Check sheet for the modelled part. Datum: model origin and axes. Units: mm. A direction names the side the tool comes from. Coordinates: 2 decimals unless noted, no trailing zeros. Write each loop counter-clockwise with the first axis right and the second up, starting at its lowest first coordinate (ties: lowest second). Pieces come first, ordered by that corner, then holes. Notation, with made-up numbers: (78.25, -3.5) - (135.25, -3.5) arc R8 ccw to (135.25, 8.5) - close; hole circle Ø3 at (25.25, -27). An arc over 180 degrees is marked (long way). Answer as CSV lines item,"result". Start each with the question number.
Autodesk Inventor part; units mm, degrees
ref_plane "Work Plane1" through (-73, 67.0488, 53) normal (0, -0.2132164, 0.977005) x (1, 0, 0)
ref_plane "YZ Plane" through (0, 0, 0) normal (1, 0, 0) x (0, 1, 0)
ref_plane "XZ Plane" through (0, 0, 0) normal (0, 1, 0) x (-1, 0, 0)
sketch "Sketch1" plane through (0, 0, 0) normal (0, 0, 1) x (1, 0, 0)
  line L0 (-75, 67.0488) -> (75, 67.0488)
  arc A0 (-75, -67.9512) -> (-48.2091, -125.4046) centre (0, -67.9512) ccw
  arc A1 (48.2091, -125.4046) -> (75, -67.9512) centre (0, -67.9512) ccw
  arc A2 (32.1394, -106.2534) -> (-32.1394, -106.2534) centre (0, -67.9512) ccw
  line L1 (-48.2091, -125.4046) -> (-32.1394, -106.2534) construction
  line L2 (-32.1394, -106.2534) -> (0, -67.9512) construction
  line L3 (-48.2091, -125.4046) -> (-32.1394, -106.2534) construction
  line L4 (75, -67.9512) -> (75, 67.0488)
  line L5 (-75, -67.9512) -> (-75, 67.0488)
  line L6 (0, -67.9512) -> (0, -148.7803) construction
  line L7 (-32.1394, -106.2534) -> (-48.2091, -125.4046)
  line L8 (48.2091, -125.4046) -> (32.1394, -106.2534)
  point P0 (0, 0)
  dimension "d0" = 150
  dimension "d2" = 135
  dimension "d3" = 135
  dimension "d7" = 135
  dimension "d8" = 50
  dimension "d19" = 75
  dimension "d25" = 75
  dimension "d26" = 0
  dimension "d29" = 50
  dimension "d31" = 50
  dimension "d34" = 40
  dimension "d35" = 40
extrude "Extrusion1" add sketch "Sketch1" along normal blind 3
sketch "Sketch5" plane through (0, 0, 3) normal (0, 0, 1) x (1, 0, 0)
  arc A0 (32.1394, -106.2534) -> (-32.1394, -106.2534) centre (0, -67.9512) ccw
  line L0 (32.1394, -106.2534) -> (48.2091, -125.4046)
  line L1 (-48.2091, -125.4046) -> (-32.1394, -106.2534)
  arc A1 (37.2817, -112.3818) -> (-37.2817, -112.3818) centre (0, -67.9512) ccw
  arc A2 (32.1394, -106.2534) -> (-32.1394, -106.2534) centre (0, -67.9512) ccw
  arc A3 (32.1394, -106.2534) -> (-32.1394, -106.2534) centre (0, -67.9512) ccw
  arc A4 (41.7812, -117.7441) -> (-41.7812, -117.7441) centre (0, -67.9512) ccw
  arc A5 (46.2807, -123.1064) -> (-46.2807, -123.1064) centre (0, -67.9512) ccw
  line L2 (-46.2807, -123.1064) -> (-41.7812, -117.7441)
  line L3 (-37.2817, -112.3818) -> (-32.1394, -106.2534)
  line L4 (32.1394, -106.2534) -> (37.2817, -112.3818)
  line L5 (41.7812, -117.7441) -> (46.2807, -123.1064)
  point P0 (0, 0)
  dimension "d49" = 58
  dimension "d52" = 65
  dimension "d53" = 72
extrude "Extrusion3" add sketch "Sketch5" along normal blind 8 contours A0 L1 A1 L0 | A4 L1 A5 L0
sketch "Sketch7" plane through (-48.2091, -125.4046, 3) normal (0.7660444, -0.6427876, 0) x (0, 0, -1)
  line L0 (0, 10) -> (-8, 10)
  line L1 (-4.5, 10) -> (0, 10)
  line L2 (0, 10) -> (0, 17)
  line L3 (0, 10) -> (0, 17)
  line L4 (0, 17) -> (-4.5, 17)
  line L5 (0, 17) -> (-8, 17)
  arc A0 (-4.5, 10) -> (-4.5, 17) centre (-4.5, 13.5) ccw
  line L6 (-19.076, 75) -> (19.2246, 75) construction
  point P0 (3, 127.0537)
  dimension "d58" = 4.5
  dimension "d59" = 0
  dimension "d60" = 0
  dimension "d61" = 3.5
  dimension "d62" = 58
revolve "Revolution1" add sketch "Sketch7" angle 280 about axis through (0, -67.9512, 22.076) along (0, 0, -1)
sketch "Sketch18" plane through (0, 0, 0) normal (0, 0, -1) x (-1, 0, 0)
  arc A0 (32.1394, -106.2534) -> (-32.1394, -106.2534) centre (0, -67.9512) ccw
  line L0 (32.1394, -106.2534) -> (48.2091, -125.4046)
  arc A1 (32.1394, -106.2534) -> (-32.1394, -106.2534) centre (0, -67.9512) ccw
  line L1 (-32.1394, -106.2534) -> (-47.5756, -125.4046)
  line L2 (32.1394, -106.2534) -> (48.2091, -125.4046)
  line L3 (75, 67.0488) -> (-75, 67.0488)
  line L4 (-75, 67.0488) -> (-75, -67.9512)
  arc A2 (-75, -67.9512) -> (-48.2091, -125.4046) centre (0, -67.9512) ccw
  line L5 (-48.2091, -125.4046) -> (-32.1394, -106.2534)
  arc A3 (32.1394, -106.2534) -> (-32.1394, -106.2534) centre (0, -67.9512) ccw
  line L6 (32.1394, -106.2534) -> (48.2091, -125.4046)
  arc A4 (48.2091, -125.4046) -> (75, -67.9512) centre (0, -67.9512) ccw
  line L7 (75, -67.9512) -> (75, 67.0488)
  arc A5 (-75, -67.9512) -> (-48.2091, -125.4046) centre (0, -67.9512) ccw
  line L8 (-75, -67.9512) -> (-75, 67.0488)
  line L9 (75, -67.9512) -> (75, 67.0488)
  line L10 (75, 67.0488) -> (75, -67.9512)
  arc A6 (-75, -67.9512) -> (-48.2091, -125.4046) centre (0, -67.9512) ccw
  arc A7 (48.2091, -125.4046) -> (75, -67.9512) centre (0, -67.9512) ccw
  arc A8 (48.2091, -125.4046) -> (75, -67.9512) centre (0, -67.9512) ccw
  arc A9 (35.4639, -107.3379) -> (-35.4639, -107.3379) centre (0, -67.9512) ccw
  line L11 (0, -67.9512) -> (35.4639, -107.3379) construction
  line L12 (0, -67.9512) -> (-35.4639, -107.3379) construction
  line L13 (0, -67.9512) -> (0, -163.7516) construction
  arc A10 (46.2807, -123.1064) -> (-46.2807, -123.1064) centre (0, -67.9512) ccw construction
  line L14 (72, -67.9512) -> (72, 64.0488)
  line L15 (72, 64.0488) -> (-72, 64.0488)
  line L16 (-72, 64.0488) -> (-72, -67.9512)
  arc A11 (-72, -67.9512) -> (-48.1774, -121.4576) centre (0, -67.9512) ccw
  arc A12 (48.1774, -121.4576) -> (72, -67.9512) centre (0, -67.9512) ccw
  line L17 (-48.1774, -121.4576) -> (-35.4639, -107.3379)
  line L18 (35.4639, -107.3379) -> (48.1774, -121.4576)
  point P0 (0, 0)
  dimension "d99" = 84
  dimension "d100" = 42
  dimension "d101" = 53
  dimension "d102" = 3
  dimension "d103" = 3
extrude "Extrusion8" add sketch "Sketch18" against normal blind 53
sketch "Sketch19" plane through (75, -67.9512, 0) normal (1, 0, 0) x (0, 0, -1)
  line L0 (-3, 132) -> (-3, 0)
  line L1 (-3, 0) -> (-3, 0)
  line L2 (-3, 0) -> (-3, 132)
  line L3 (-11, 0) -> (-11, -53.5064)
  line L4 (-53, 0) -> (-53, 135)
  line L5 (-53, 0) -> (-53, -57.4533)
  line L6 (0, -57.4533) -> (-53, -57.4533)
  line L7 (-53, 135) -> (-53, -57.4533)
  line L8 (-53, -57.4533) -> (-11, -57.4533)
  line L9 (0, 135) -> (-53, 135)
  line L10 (-11, -57.4533) -> (-53, 135)
  point P0 (0, 67.9512)
  dimension "d106" = 0
extrude "Extrusion9" cut sketch "Sketch19" against normal blind 150
sketch "Sketch20" plane through (-32.1394, -106.2534, 15.1794) normal (0.7660444, -0.6427876, 0) x (0, 0, -1)
  ellipse E0 centre (7.6794, -11.4625) end of major axis (11.1794, -11.4625) minor radius 3.4979 (7.6794, -14.9604) -> (7.6794, -7.9647) ccw
  circle A0 centre (7.6794, -11.4625) radius 3.5
  line L0 (-25.5689, 50.0375) -> (41.9904, 50.0375) construction
  point P0 (15.1794, 102.0537)
  dimension "d109" = 61.5
revolve "Revolution4" cut sketch "Sketch20" angle 2 about axis through (0.0241, -67.9225, 40.7483) along (0, 0, -1)
mirror "Mirror3" about plane through (0, 0, 0) normal (1, 0, 0) of "Revolution4"
fillet "Fillet1" radius 2 12 edges at (75, 67.0488, 26.5) (-48.2091, -125.4046, 5.5) (-32.1394, -106.2534, 7.5897) (48.2091, -125.4046, 5.5) (32.1394, -106.2534, 7.5897) (-75, 67.0488, 26.5) (0, 67.0488, 0) (-67.9731, -99.6476, 0) (-75, -0.4512, 0) (67.9731, -99.6476, 0) (75, -0.4512, 0) (0, -17.9512, 0)
sketch "Sketch23" plane through (0, 0, 0) normal (0, 0, -1) x (-1, 0, 0)
  arc A0 (43.4935, -116.2556) -> (-43.4935, -116.2556) centre (0, -67.9512) ccw
  line L0 (0, -67.9512) -> (0, -128.8082) construction
  arc A1 (43.4935, -116.2556) -> (-43.4935, -116.2556) centre (0, -67.9512) ccw
  line L1 (-56.2917, -100.4512) -> (-50.2295, -96.9512) construction
  line L2 (0, -67.9512) -> (-50.2295, -96.9512) construction
  line L3 (-56.2917, -100.4512) -> (0, -67.9512) construction
  circle A2 centre (-55.0106, -95.6701) radius 3.5 construction
  line L4 (-59.6154, -93.8549) -> (-53.1953, -91.0653) construction
  arc A3 (38.8096, -111.0536) -> (-38.8096, -111.0536) centre (0, -67.9512) ccw construction
  arc A4 (-62.3186, -49.4745) -> (-59.6154, -93.8549) centre (0, -67.9512) ccw construction
  line L5 (0, -67.9512) -> (-62.3186, -49.4745) construction
  line L6 (0, -67.9512) -> (-59.6154, -93.8549) construction
  arc A5 (35.4639, -107.3379) -> (-35.4639, -107.3379) centre (0, -67.9512) ccw construction
  arc A6 (-55.6074, -51.4643) -> (-53.1953, -91.0653) centre (0, -67.9512) ccw construction
  line L7 (0, -67.9512) -> (-55.6074, -51.4643) construction
  line L8 (0, -67.9512) -> (-53.1953, -91.0653) construction
  line L9 (-62.3186, -49.4745) -> (-55.6074, -51.4643)
  arc A7 (-62.3186, -49.4745) -> (-56.2917, -100.4512) centre (0, -67.9512) ccw
  arc A8 (-55.6074, -51.4643) -> (-50.2295, -96.9512) centre (0, -67.9512) ccw
  line L10 (-56.2917, -100.4512) -> (-50.2295, -96.9512)
  point P0 (0, 0)
  dimension "d113" = 7
  dimension "d114" = 60
  dimension "d115" = 7
  dimension "d116" = 7
  dimension "d117" = 40
  dimension "d118" = 40
extrude "Extrusion10" cut sketch "Sketch23" against normal up to next
sketch "Sketch24" plane through (-73, 67.0488, 53) normal (0, -0.2132164, 0.977005) x (1, 0, 0)
  line L0 (146, 0) -> (0, 0)
  ellipse E0 centre (0, -2.0471) end of major axis (0, 0) minor radius 2 (0, 0) -> (-2, -2.0471) ccw
  line L1 (-2, -138.1774) -> (-2, -2.0471)
  ellipse E1 centre (73, -138.1774) end of major axis (73, -61.4122) minor radius 75 (-2, -138.1774) -> (23.235, -195.609) ccw
  ellipse E2 centre (24.562, -194.0775) end of major axis (24.562, -196.1246) minor radius 2 (23.235, -195.609) -> (26.0941, -195.3933) ccw
  line L2 (39.5998, -178.9191) -> (26.0941, -195.3933)
  ellipse E3 centre (38.0677, -177.6032) end of major axis (38.0677, -175.5562) minor radius 2 (39.5998, -178.9191) -> (39.4112, -176.0869) ccw
  ellipse E4 centre (73, -138.1774) end of major axis (73, -189.3542) minor radius 50 (106.5888, -176.0869) -> (39.4112, -176.0869) ccw
  ellipse E5 centre (107.9323, -177.6032) end of major axis (107.9323, -175.5562) minor radius 2 (106.5888, -176.0869) -> (106.4002, -178.9191) ccw
  line L3 (119.9059, -195.3933) -> (106.4002, -178.9191)
  ellipse E6 centre (121.438, -194.0775) end of major axis (121.438, -196.1246) minor radius 2 (119.9059, -195.3933) -> (122.765, -195.609) ccw
  ellipse E7 centre (73, -138.1774) end of major axis (73, -61.4122) minor radius 75 (122.765, -195.609) -> (148, -138.1774) ccw
  line L4 (148, -2.0471) -> (148, -138.1774)
  ellipse E8 centre (146, -2.0471) end of major axis (146, 0) minor radius 2 (148, -2.0471) -> (146, 0) ccw
  point P0 (73, -76.8075)
extrude "Extrusion11" add sketch "Sketch24" along normal blind 3
ref_plane "Work Plane1" through (-73, 67.0488, 53) normal (0, -0.2132164, 0.977005) x (1, 0, 0)
split "Split1" plane through (-73, 67.0488, 53) removes the side toward (0, 0.2132164, -0.977005)
sketch "Sketch25" plane through (-73, 66.4091, 55.931) normal (0, -0.2132164, 0.977005) x (1, 0, 0)
  circle A0 centre (88, -40) radius 5
  line L0 (146, 0) -> (0, 0)
  line L1 (148, -138.1774) -> (148, -2.0471)
  point P0 (73, -76.8075)
  dimension "d124" = 10
  dimension "d125" = 40
  dimension "d126" = 60
extrude "Extrusion12" cut sketch "Sketch25" against normal blind 10
sketch "Sketch26" plane through (-73, 66.4091, 55.931) normal (0, -0.2132164, 0.977005) x (1, 0, 0)
  circle A0 centre (4, -6.071) radius 1.25
  circle A1 centre (4, -93.071) radius 1.25
  circle A2 centre (142, -93.071) radius 1.25
  circle A3 centre (142, -6.071) radius 1.25
  line L0 (146, 0) -> (0, 0)
  line L1 (-2, -2.0471) -> (-2, -138.1774)
  line L2 (148, -138.1774) -> (148, -2.0471)
  point P0 (73, -76.8075)
  dimension "d129" = 2.5
  dimension "d130" = 2.5
  dimension "d131" = 2.5
  dimension "d132" = 2.5
  dimension "d133" = 6.071
  dimension "d134" = 6.071
  dimension "d135" = 6
  dimension "d136" = 6
  dimension "d137" = 6
  dimension "d138" = 6
  dimension "d139" = 93.071
  dimension "d140" = 93.071
extrude "Extrusion13" cut sketch "Sketch26" against normal up to next
properties part number "Lock Base"
(1) Tool access check on faces 4 (the face through (-40.06, -116.01, 14.56)), 5 (the face through (-1.05, -6.77, 39.96)). Record the directions out of +Z, -Z, +X, -X, +Y, -Y that give a thin tool (end or side, any length) a straight path to the whole face; none if there is none.
(2) Release check for a two-part mould opening along X. For faces 1 (the face through (40.248, -116.232, 14.516)), 2 (the face through (-75, -3, 39)), 3 (the face through (-1.05, -6.13, 37.03)) record: pulls with the +X half, pulls with the -X half, needs draft (parallel to the pull), parting line crosses it, or undercut.
(3) Cross-section at B-B on y = -15.5. Record the boundary of the cut face in (x, z), plus the area to 3 significant figures.
(4) Material ranges on probe 1 along Z at (x, y) = (4, 45.5); probe 2 along Z at (x, y) = (27, -25.5), recorded low to high. Write a range as from..to.
(5) Go/stop test with flat-tipped pins: P1, Ø1.5, axis at x = -15.5, y = 8.5, coming from the -Z side; P2, Ø10, axis at y = -83.5, z = 30, coming from the -X side; P3, Ø6, axis at x = -11.5, y = -5.5, coming from the -Z side; P4, Ø5, axis at x = 40.5, y = -34, coming from the -Z side. Record where each tip stops, or that it passes through.
(6) Cross-section at A-A on z = 40. Record the boundary of the cut face in (x, y), plus the area to 3 significant figures.
Checked values:
1,face 4,"-Z, -Y"
1,face 5,"+Z, +X, -X, -Y"
2,face 1,"undercut"
2,face 2,"pulls with the -X half"
2,face 3,"needs draft"
3,outline,"(-75, 34.98) - (75, 34.98) - (75, 38.06) - (-75, 38.06) - close"
3,area,"461 mm^2"
4,probe 1,"48.3..51.37"
4,probe 2,"32.8..35.87"
5,P1,"z = 40.06"
5,P2,"through"
5,P3,"z = 36.51"
5,P4,"z = 30.4"
6,outline,"(-75, -6.59) - (75, -6.59) - (75, 7.48) - (-75, 7.48) - close"
6,area,"2,110 mm^2"
